Design review of the part shown in the three views and the two pictorial views. Dimensions are in mm from the part's minimum x, y and z. A direction names the side the tool comes from. Round coordinates to 2 decimals unless told otherwise and drop trailing zeros. Order: outer loops, then holes, each group sorted by start corner. A loop starts at its lowest first (then second) coordinate and runs counter-clockwise, first axis right, second up.
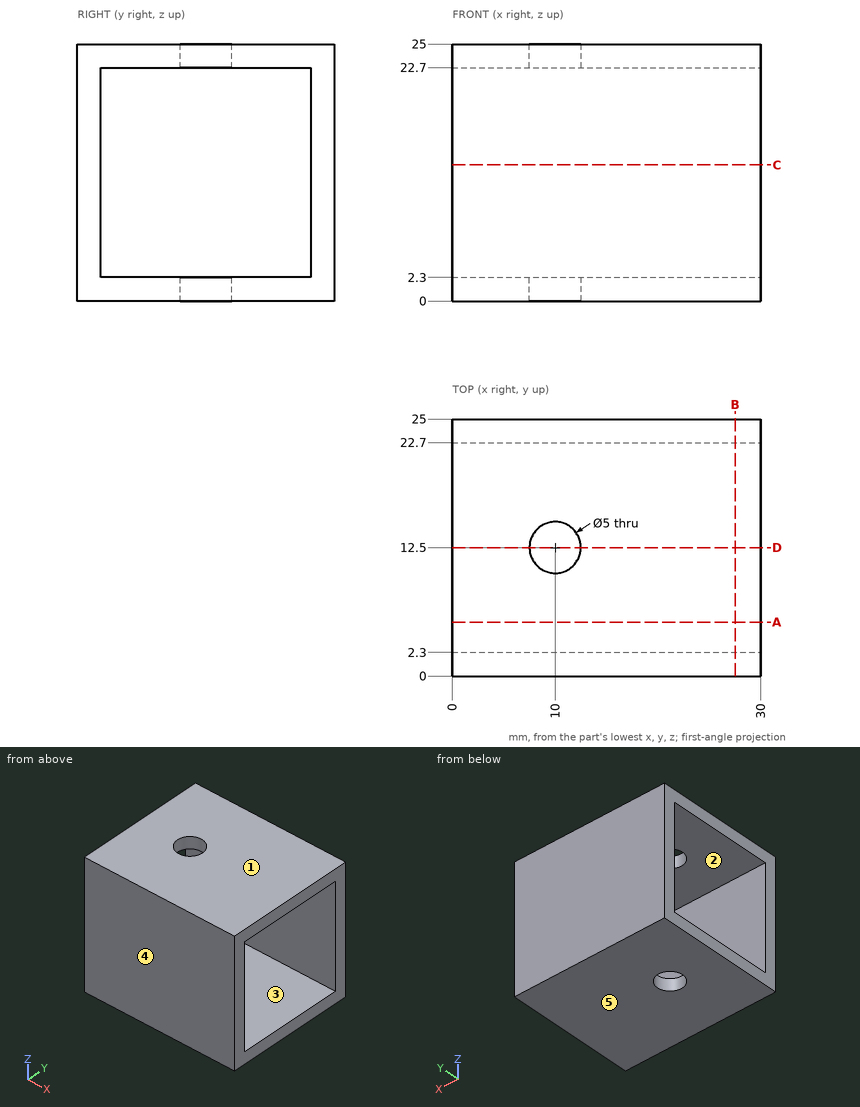
1) For the marked faces 1 and 2, list the 3-axis set-ups (+Z, -Z, +X, -X, +Y, -Y) from which the entire face can be reached by the end or side of a thin tool; tool diameter is ignored.
Results:
face 1: +Z, +X, -X, +Y, -Y
face 2: +X, -X
2) Take a section at B-B on x = 27.5. Give the boundary of the cut face in (y, z), plus the area to 3 significant figures.
Results:
outline: (0, 0) - (25, 0) - (25, 25) - (0, 25) - close; hole (2.3, 2.3) - (22.7, 2.3) - (22.7, 22.7) - (2.3, 22.7) - close
area: 209 mm2
3) The part is to be moulded in two halves that separate along Z. For the marked faces 3, 4 and 5, say which applies: released by +Z, released by -Z, zero draft, split by the parting line, or undercut.
Results:
face 3: undercut
face 4: zero draft
face 5: released by -Z
4) Take a section at D-D on y = 12.5. Give the boundary of the cut face in (x, z).
Results:
outline: (0, 0) - (7.5, 0) - (7.5, 2.3) - (0, 2.3) - close; (0, 22.7) - (7.5, 22.7) - (7.5, 25) - (0, 25) - close; (12.5, 0) - (30, 0) - (30, 2.3) - (12.5, 2.3) - close; (12.5, 22.7) - (30, 22.7) - (30, 25) - (12.5, 25) - close
5) Take a section at A-A on y = 5.25. Give the boundary of the cut face in (x, z).
Results:
outline: (0, 0) - (30, 0) - (30, 2.3) - (0, 2.3) - close; (0, 22.7) - (30, 22.7) - (30, 25) - (0, 25) - close
6) Clearance check with a flat-ended pin moving along its axis: P1, Ø8, axis at y = 16.5, z = 17.5, coming from the -X side. State where the tip first meets the part, or that it passes through.
Results:
P1: passes through
7) To check wall thickness, follow line 1 along Y through (x, z) = (17.5, 9); line 2 along Y through (x, z) = (10, 23.45). State the ranges of each line that lie inside material, in increasing order.
Results:
line 1: y = 0 to 2.3, 22.7 to 25
line 2: y = 0 to 10, 15 to 25
